Geometry check sheet. Reference: drawing and pictorial views, mm from the part's lowest x, y, z. A direction names the side the tool comes from. Round coordinates to 2 decimals unless told otherwise and drop trailing zeros. Write each loop counter-clockwise with the first axis right and the second up, starting at its lowest first coordinate (ties: lowest second). Pieces come first, ordered by that corner, then holes. Notation, with made-up numbers: (77, -39) -> (114, -39) arc R20 ccw to (114, -28) -> close; hole circle Ø3 at (63, 70). An arc over 180 degrees is marked (long way). Answer as a JSON object with one key per item and string values. Group by question number.
(1) Scan lines: L1, parallel to X at y = 84, z = 38; L2, parallel to Z at x = 292, y = 11 (1 decimal); L3, parallel to Z at x = 50.8, y = 86.5. Record each from-to range of solid material in increasing order. Write a range as from..to.
(2) Gauge pin test, flat ends, axial feed: pin 1 Ø10.5 at (x, z) = (284, 3.5) entering from +Y; pin 2 Ø5.5 at (y, z) = (78.5, 24) entering from +X; pin 3 Ø24 at (x, z) = (137.5, 39) entering from -Y (1 decimal). Record the tip position at first contact, or that the pin passes through.
(3) Sectioned sample at C-C on z = 5. Record the cut outline in (x, y).
(4) Sectioned sample at B-B on z = 38.1. Count the separate pieces of the cut face and the enclosed holes in it, and give its area (3 significant figures).
(5) Set-up check for the marked faces 1 and 2: record each of +Z, -Z, +X, -X, +Y, -Y from which the full face is reachable in a straight line by a thin tool's end or side.
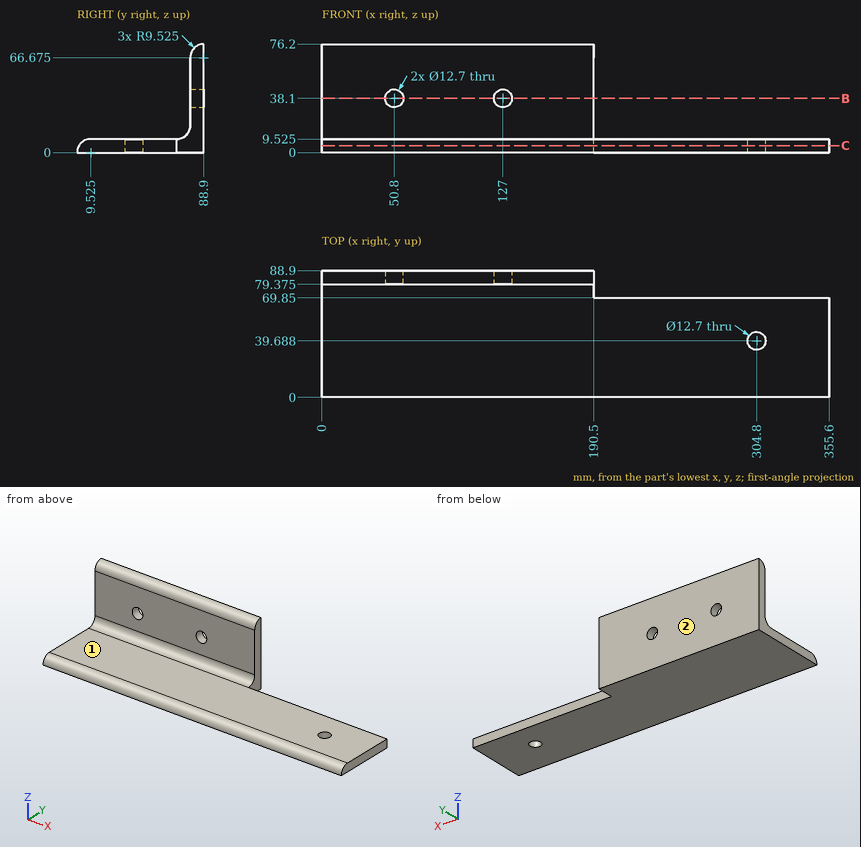
Computed values:
{
 "1": {"L1": "0..44.45, 57.15..120.65, 133.35..190.5", "L2": "0..9.5", "L3": "0..31.75, 44.45..75.89"},
 "2": {"pin 1": "y = 69.85", "pin 2": "x = 190.5", "pin 3": "y = 79.4"},
 "3": {"outline": "(0, 1.42) -> (355.6, 1.42) -> (355.6, 69.85) -> (190.5, 69.85) -> (190.5, 88.9) -> (0, 88.9) -> close; hole circle Ø12.7 at (304.8, 39.69)"},
 "4": {"separate pieces": "3", "enclosed holes": "0", "area": "1,570 mm2"},
 "5": {"face 1": "+Z, +X, -X, -Y", "face 2": "+Z, -Z, +X, -X, +Y"}
}
